Read the model definition and answer for the solid it produces. Units are mm, in the model's axes. A direction names the side the tool comes from. Give positions to 0.01 mm unless a question says otherwise; leave off trailing zeros. Use a Markdown table: item, result.
from build123d import *

# Parameters (mm, degrees)
SKETCH072_R          = 1.65
SKETCH072_W          = 30
SKETCH072_H          = 38
PAD031_DEPTH         = 5
SKETCH073_W          = 33
SKETCH073_H          = 41
SKETCH073_W_2        = 30
SKETCH073_H_2        = 38
PAD032_DEPTH         = 18
SKETCH108_W          = 33
SKETCH108_H          = 41
PAD049_DEPTH         = 1.5
POCKET055_DEPTH      = 41.001
POCKET056_DEPTH      = 50
POCKET056_DEPTH_BACK = 5


with BuildPart() as part:
    # Sketch072 → Pad031 (new body)
    with BuildSketch(Plane.XY):
        with BuildLine():
            Line((16.5, 59.5), (-16.5, 59.5))
            Line((-16.5, 59.5), (-16.5, 46.25))
            ThreePointArc((-20, 42.75), (-17.525126, 43.775126), (-16.5, 46.25))
            ThreePointArc((-20, 42.75), (-23.75, 39), (-20, 35.25))
            ThreePointArc((-16.5, 31.75), (-17.525126, 34.224874), (-20, 35.25))
            Line((-16.5, 18.5), (-16.5, 31.75))
            Line((16.5, 18.5), (-16.5, 18.5))
            Line((16.5, 18.5), (16.5, 31.75))
            ThreePointArc((20, 35.25), (17.525126, 34.224874), (16.5, 31.75))
            ThreePointArc((20, 35.25), (23.75, 39), (20, 42.75))
            ThreePointArc((16.5, 46.25), (17.525126, 43.775126), (20, 42.75))
            Line((16.5, 59.5), (16.5, 46.25))
        make_face()
        with Locations((20, 39)):
            Circle(SKETCH072_R, mode=Mode.SUBTRACT)
        with Locations((-20, 39)):
            Circle(SKETCH072_R, mode=Mode.SUBTRACT)
        with Locations((0, 39)):
            Rectangle(SKETCH072_W, SKETCH072_H, mode=Mode.SUBTRACT)
    extrude(amount=-PAD031_DEPTH)

    # Sketch073 (on Face20 of Pad031) → Pad032 (join)
    with BuildSketch(Plane(origin=(0, 0, -5), x_dir=(1, 0, 0), z_dir=(0, 0, -1))):
        with Locations((0, -39)):
            Rectangle(SKETCH073_W, SKETCH073_H)
        with Locations((0, -39)):
            Rectangle(SKETCH073_W_2, SKETCH073_H_2, mode=Mode.SUBTRACT)
    extrude(amount=PAD032_DEPTH)

    # Sketch108 (on Face23 of Pad032) → Pad049 (join)
    with BuildSketch(Plane(origin=(0, 0, -23), x_dir=(1, 0, 0), z_dir=(0, 0, -1))):
        with Locations((0, -39)):
            Rectangle(SKETCH108_W, SKETCH108_H)
        Polygon((0, -40.613829), (-13.725924, -58), (13.725924, -58), align=None, mode=Mode.SUBTRACT)
        Polygon((15, -56.386171), (1.274076, -39), (15, -21.613829), align=None, mode=Mode.SUBTRACT)
        Polygon((13.725924, -20), (-13.725924, -20), (0, -37.386171), align=None, mode=Mode.SUBTRACT)
        Polygon((-1.274076, -39), (-15, -21.613829), (-15, -56.386171), align=None, mode=Mode.SUBTRACT)
    extrude(amount=PAD049_DEPTH)

    # Sketch109 (on Face5 of Pad049) → Pocket055 (cut, through all)
    with BuildSketch(Plane(origin=(0, 59.5, 0), x_dir=(-1, 0, 0), z_dir=(0, 1, 0))):
        Polygon((-15, -2.730289), (-15, -21.769711), (-1.716682, -12.25), align=None)
        Polygon((1.716682, -12.25), (15, -21.769711), (15, -2.730289), align=None)
        Polygon((-13.283318, -23), (13.283318, -23), (0, -13.480289), align=None)
        Polygon((-13.283318, -1.5), (13.283318, -1.5), (0, -11.019711), align=None)
    extrude(amount=-POCKET055_DEPTH, mode=Mode.SUBTRACT)

    # Sketch110 (on Face28 of Pocket055) → Pocket056 (cut, two sides)
    with BuildSketch(Plane(origin=(-16.5, 0, 0), x_dir=(0, -1, 0), z_dir=(-1, 0, 0))) as pocket056_sk:
        Polygon((-56.473161, -23), (-47.386076, -14.611922), (-39.778284, -23), align=None)
        Polygon((-58, -21.687574), (-58, -3.06762), (-48.807871, -13.202532), align=None)
        with BuildLine():
            Line((-56.721716, -1.5), (-47.386076, -11.793142))
            Line((-47.386076, -11.793142), (-40.026839, -5))
            Line((-40.026839, -5), (-44.75, -5))
            ThreePointArc((-46.25, -3.5), (-45.81066, -4.56066), (-44.75, -5))
            Line((-46.25, -1.5), (-46.25, -3.5))
            Line((-46.25, -1.5), (-56.721716, -1.5))
        make_face()
        with BuildLine():
            Line((-36.934247, -5), (-30.06962, -11.679097))
            Line((-30.06962, -11.679097), (-21.310863, -1.5))
            Line((-21.310863, -1.5), (-31.75, -1.5))
            Line((-31.75, -1.5), (-31.75, -3.5))
            ThreePointArc((-33.25, -5), (-32.18934, -4.56066), (-31.75, -3.5))
            Line((-36.934247, -5), (-33.25, -5))
        make_face()
        Polygon((-28.741998, -13.202532), (-20, -3.042912), (-20, -21.70826), align=None)
        Polygon((-37.210398, -23), (-30.06962, -14.701258), (-21.540358, -23), align=None)
        Polygon((-38.5, -21.43238), (-31.418503, -13.202532), (-38.5, -6.312426), (-45.964281, -13.202532), align=None)
    extrude(amount=-POCKET056_DEPTH, mode=Mode.SUBTRACT)
    extrude(pocket056_sk.sketch, amount=POCKET056_DEPTH_BACK, mode=Mode.SUBTRACT)


with BuildPart() as part_1:
    # Body023 placement: moved
    add(part.part.moved(Location((0, 0, 32))))


solid = part_1.part
Item 1: For a pull along Z with two mould halves and no side action, classify faces 4 (the face through (0, 59.5, 19)), 5 (the face through (-6.735, 58.76, 25.807)) as +Z half, -Z half, draft (parallel to the pull), parting line (faces both ways), or undercut.
Return value:
| item | result |
|---|---|
| face 4 | draft |
| face 5 | undercut |
Item 2: Each of these flat-tipped pins is pushed along its axis until it touches: P1, Ø8, axis at y = 29.5, z = 28.5, coming from the +X side; P2, Ø7.5, axis at y = 45.5, z = 15.5, coming from the -X side; P3, Ø4.5, axis at x = 20, y = 39, coming from the -Z side. Where does it stop, or does it pass through?
Return value:
| item | result |
|---|---|
| P1 | x = 16.97 |
| P2 | x = -16.5 |
| P3 | z = 27 |
Item 3: A cutting plane is placed at A-A (x = 10.5). Count the separate pieces of the cut face and the enclosed holes in it, then the cut area to 3 significant figures.
Return value:
| item | result |
|---|---|
| separate pieces | 10 |
| enclosed holes | 0 |
| area | 33.4 mm^2 |
Item 4: A tool of negligible diameter and unlimited length cuts with its end or side. For faces 1 (the face through (-8.451, 58.76, 24.576)), 2 (the face through (17.5, 43.8, 29.5)), 3 (the face through (16, 51, 30.5)), from which of +Z, -Z, +X, -X, +Y, -Y can it reach the whole face along a straight path? Write none if from no direction.
Return value:
| item | result |
|---|---|
| face 1 | +Y, -Y |
| face 2 | +Z, -Z, +X, +Y |
| face 3 | +X, -X |
Item 5: Straight lines are drawn through the part: line 1 along Y through (x, z) = (-20, 30.4); line 2 along Y through (x, z) = (15.5, 13.5); line 3 along Y through (x, z) = (1, 21.25). For each, find the intervals that lie inside material, in ascending order. Write a range as [from, to].
Return value:
| item | result |
|---|---|
| line 1 | [35.25, 37.35], [40.65, 42.75] |
| line 2 | [18.5, 20], [23.3, 26.17], [33.34, 35.98], [41.16, 43.86], [51.6, 54.55], [58, 59.5] |
| line 3 | [18.5, 20], [58, 59.5] |
